from build123d import *

# Parameters (mm, degrees)
SKETCH1_R           = 60
SKETCH1_R_2         = 45
BOSS_EXTRUDE1_DEPTH = 5
SKETCH2_R           = 45
SKETCH2_R_2         = 40
BOSS_EXTRUDE2_DEPTH = 56
SKETCH3_R           = 40
SKETCH3_R_2         = 3.75
BOSS_EXTRUDE3_DEPTH = 10


with BuildPart() as part:
    # Sketch1 → Boss-Extrude1 (new body)
    with BuildSketch(Plane(origin=(0, 0, 0), x_dir=(1, 0, 0), z_dir=(0, 1, 0))):
        Circle(SKETCH1_R)
        Circle(SKETCH1_R_2, mode=Mode.SUBTRACT)
    extrude(amount=BOSS_EXTRUDE1_DEPTH)

    # Sketch2 → Boss-Extrude2 (add)
    with BuildSketch(Plane(origin=(0, 0, 0), x_dir=(1, 0, 0), z_dir=(0, 1, 0))):
        Circle(SKETCH2_R)
        Circle(SKETCH2_R_2, mode=Mode.SUBTRACT)
    extrude(amount=BOSS_EXTRUDE2_DEPTH)

    # Sketch3 → Boss-Extrude3 (add)
    with BuildSketch(Plane(origin=(0, 56, 0), x_dir=(1, 0, 0), z_dir=(0, 1, 0))):
        Circle(SKETCH3_R)
        Circle(SKETCH3_R_2, mode=Mode.SUBTRACT)
    extrude(amount=-BOSS_EXTRUDE3_DEPTH)


solid = part.part
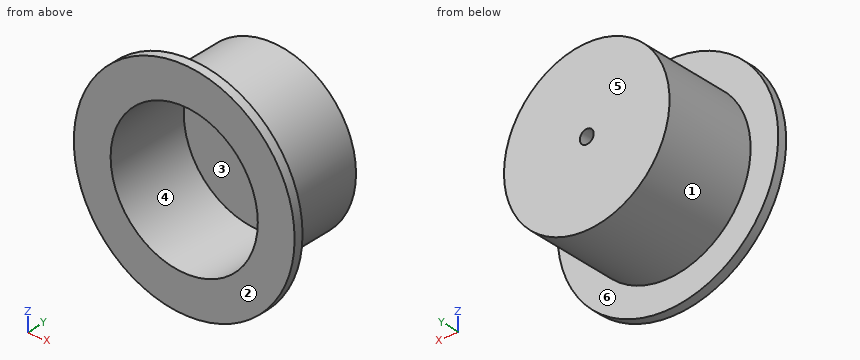
Can you work these out from the model? Positions are in its coordinate system, mm. Face numbers are marked on the shaded views. A direction names the side the tool comes from. Give positions to 0.01 mm unless a question says otherwise; leave off trailing zeros. Write each loop counter-clockwise with the first axis right and the second up, starting at its lowest first coordinate (ties: lowest second). Pieces come first, ordered by that corner, then holes. Notation, with made-up numbers: (-19, 68.5) -> (37, 68.5) arc R28 ccw to (37, 106.5) -> close; hole circle Ø3 at (60, 31.5). An arc over 180 degrees is marked (long way). Answer as a JSON object with one key per item and string values. Group by question number.
Item 1: Suppose I cut it at B-B (x = 0). Please give me the cut outline in (y, z).
Item 2: Suppose I cut it at A-A (z = 0). Please give me the cut outline in (x, y), plus the area to 4 significant figures.
Item 3: I'm going to push flat-ended pins straight in: P1, Ø6, axis at x = 0, z = 0, coming from the +Y side; P2, Ø5, axis at y = 26.5, z = 16.5, coming from the -X side; P3, Ø1, axis at x = -38.5, y = 41.5, coming from the +Z side; P4, Ø8, axis at y = 46.5, z = 7.5, coming from the -X side. Where does each tip first touch, or does it pass through?
Item 4: We'd pull the mould along X, two halves only. Please class the marked faces 1, 2, 3 and 4: +X half, -X half, draft (parallel to the pull), parting line (faces both ways), or undercut.
Item 5: For the marked faces 5 and 6, which set-ups out of +Z, -Z, +X, -X, +Y, -Y let a thin tool reach every point of the face, with its end or its side?
Item 6: Please list where these lines run through material, in increasing order: line 1 (X direction, y = 49, z = 0); line 2 (Z direction, x = 0, y = 26.5). Write a range as [from, to].
Item 7: Suppose I cut it at C-C (y = 10.5). Please give me the cut outline in (x, z), plus the area to 3 significant figures.
Item 8: Suppose I cut it at D-D (x = 43). Please give me the cut outline in (y, z).
Findings:
{
 "1": {"outline": "(0, -60) -> (5, -60) -> (5, -45) -> (56, -45) -> (56, -3.75) -> (46, -3.75) -> (46, -40) -> (0, -40) -> close; (0, 40) -> (46, 40) -> (46, 3.75) -> (56, 3.75) -> (56, 45) -> (5, 45) -> (5, 60) -> (0, 60) -> close"},
 "2": {"outline": "(-60, 0) -> (-40, 0) -> (-40, 46) -> (-3.75, 46) -> (-3.75, 56) -> (-45, 56) -> (-45, 5) -> (-60, 5) -> close; (3.75, 46) -> (40, 46) -> (40, 0) -> (60, 0) -> (60, 5) -> (45, 5) -> (45, 56) -> (3.75, 56) -> close", "area": "1,435 mm²"},
 "3": {"P1": "passes through", "P2": "stops at x = -42.77", "P3": "stops at z = 24.1", "P4": "stops at x = -44.86"},
 "4": {"face 1": "parting line", "face 2": "draft", "face 3": "undercut", "face 4": "undercut"},
 "5": {"face 5": "+Z, -Z, +X, -X, +Y", "face 6": "+Y"},
 "6": {"line 1": "x = [-45, -3.75], [3.75, 45]", "line 2": "z = [-45, -40], [40, 45]"},
 "7": {"outline": "circle Ø90 at (0, 0); hole circle Ø80 at (0, 0)", "area": "1,340 mm²"},
 "8": {"outline": "(0, -41.84) -> (5, -41.84) -> (5, -13.27) -> (56, -13.27) -> (56, 13.27) -> (5, 13.27) -> (5, 41.84) -> (0, 41.84) -> close"}
}
